The figure shows three views and two pictorial views of one solid part (mm, origin at its lowest corner). Answer the questions. A direction names the side the tool comes from. Give positions to 0.01 mm unless a question says otherwise; leave off trailing zeros. Write each loop counter-clockwise with the first axis right and the second up, starting at its lowest first coordinate (ties: lowest second). Pieces come first, ordered by that corner, then holes. Notation, with made-up numbers: (13, 21) -> (43, 21) arc R18 ccw to (43, 55) -> close; hole circle Ø5 at (-15.75, -1). An arc over 180 degrees is marked (long way). Write item = value, one per line. Start each with the question number.
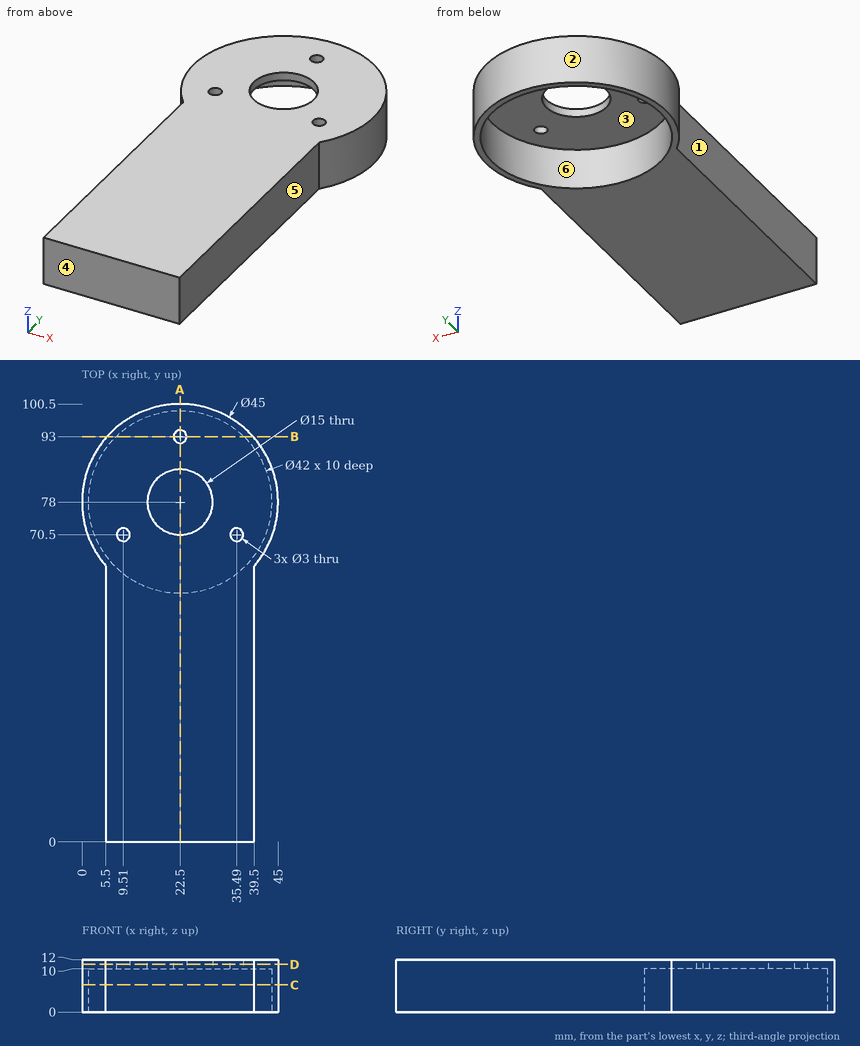
(1) A cutting plane is placed at A-A, the plane x = 22.5. Write down the section's boundary in (y, z).
(2) Find the intervals of material crossed by line 1 along Y through (x, z) = (22.5, 11.15); line 2 along Y through (x, z) = (22.5, 5.25); line 3 along Y through (x, z) = (32, 8.25) (1 decimal), in increasing order.
(3) Each of these flat-tipped pins is pushed along its axis until it touches: pin 1 (1 mm diameter, centred on y = 13.5, z = 10.5, fed in from -X); pin 2 (6 mm diameter, centred on x = 22.5, z = 5, fed in from +Y); pin 3 (6 mm diameter, centred on x = 10, y = 79, fed in from -Z). Where does it stop, or does it pass through?
(4) A cutting plane is placed at B-B, the plane y = 93. Write down the section's boundary in (x, z).
(5) Determine the mould class of the marked faces 1, 2 and 3 for opening direction Y: pulls with the +Y half, pulls with the -Y half, needs draft (parallel to the pull), parting line crosses it, or undercut.
(6) For the marked faces 4, 5 and 6, determine the directions among +Z, -Z, +X, -X, +Y, -Y from which every point of the face is accessible in a straight line to the end or side of a thin tool.
(7) A cutting plane is placed at C-C, the plane z = 6.25. Write down the section's boundary in (x, y).
(8) A cutting plane is placed at D-D, the plane z = 11. Write down the section's boundary in (x, y), then the cut area to 3 significant figures.
Results list:
q1.outline = (0, 0) -> (57, 0) -> (57, 10) -> (70.5, 10) -> (70.5, 12) -> (0, 12) -> close; (85.5, 10) -> (91.5, 10) -> (91.5, 12) -> (85.5, 12) -> close; (94.5, 10) -> (99, 10) -> (99, 0) -> (100.5, 0) -> (100.5, 12) -> (94.5, 12) -> close
q2.line_1 = 0 to 70.5, 85.5 to 91.5, 94.5 to 100.5
q2.line_2 = 0 to 57, 99 to 100.5
q2.line_3 = 0 to 59.3, 96.7 to 98.4
q3.pin_1 = 5.5
q3.pin_2 = 100.5
q3.pin_3 = 10
q4.outline = (5.73, 0) -> (7.8, 0) -> (7.8, 10) -> (21, 10) -> (21, 12) -> (5.73, 12) -> close; (24, 10) -> (37.2, 10) -> (37.2, 0) -> (39.27, 0) -> (39.27, 12) -> (24, 12) -> close
q5.face_1 = needs draft
q5.face_2 = parting line crosses it
q5.face_3 = undercut
q6.face_4 = +Z, -Z, +X, -X, -Y
q6.face_5 = +Z, -Z, +X, -Y
q6.face_6 = -Z
q7.outline = (5.5, 0) -> (39.5, 0) -> (39.5, 63.26) arc R22.5 ccw (long way) to (5.5, 63.26) -> close; hole circle Ø42 at (22.5, 78)
q8.outline = (5.5, 0) -> (39.5, 0) -> (39.5, 63.26) arc R22.5 ccw (long way) to (5.5, 63.26) -> close; hole circle Ø3 at (9.51, 70.5); hole circle Ø15 at (22.5, 78); hole circle Ø3 at (22.5, 93); hole circle Ø3 at (35.49, 70.5)
q8.area = 3,360 mm²
